Drawing for the job (mm, zero at the part's lowest x, y, z). Coordinates: 2 decimals unless noted, no trailing zeros. Write each loop counter-clockwise with the first axis right and the second up, starting at its lowest first coordinate (ties: lowest second). Pieces come first, ordered by that corner, then holes. Notation, with made-up numbers: (66, 87) -> (105, 87) arc R19 ccw to (105, 95) -> close; hole circle Ø1 at (-12, 22.5). An arc over 180 degrees is marked (long way). Write each question's results on one line, items separated by ' | '. Start each with the question number.
Q1. Drill centre lines: line 1 (Z direction, x = 23, y = 0.6); line 2 (Z direction, x = 22, y = 0.8). Where is each one in solid material? Low to high.
Q2. Saw through at A-A on z = 19. Give the cut face in (x, y).
Q3. Two-plate mould, pull along Y, no slides. Class the marked faces 1 and 2: released by +Y, released by -Y, zero draft, split by the parting line, or undercut.
Q4. Saw through at C-C on y = 0.2. Give the cut face in (x, z).
Q5. Saw through at B-B on x = 4. Give the cut face in (y, z).
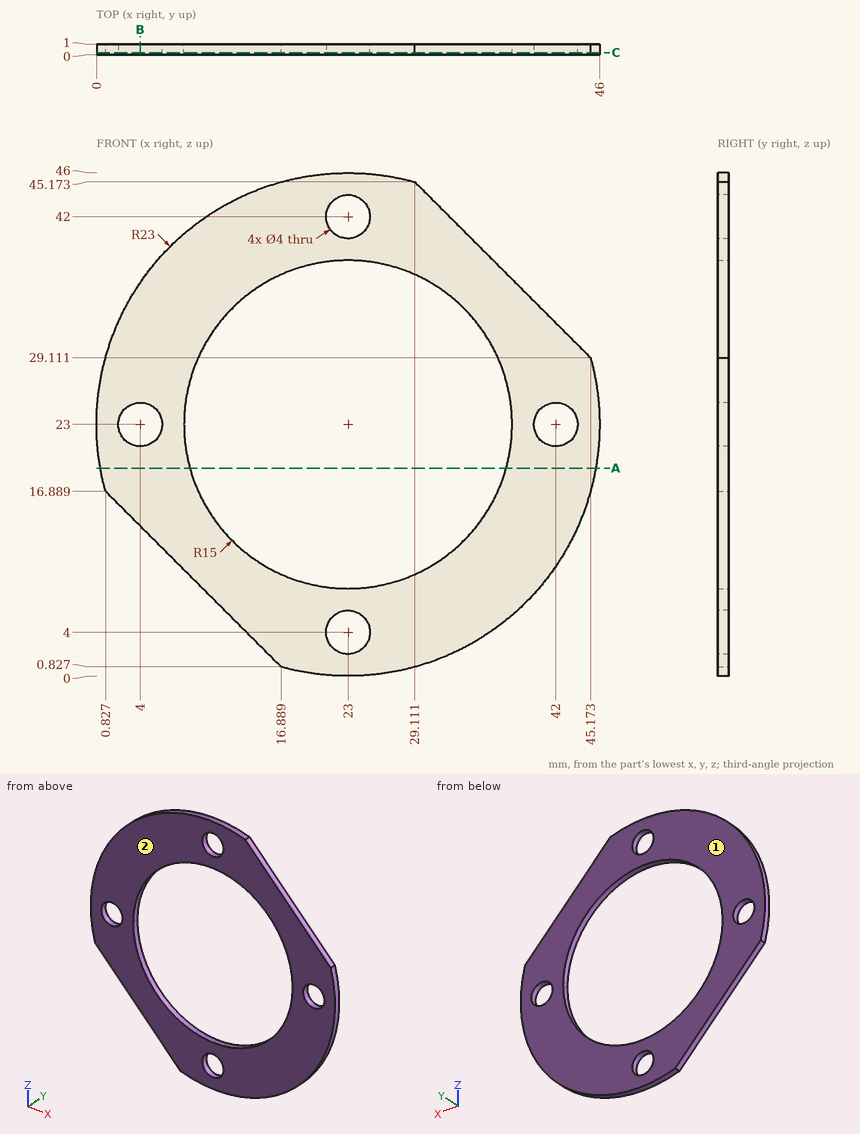
Returned:
1) line 1: z = 0 to 2, 6 to 8, 38 to 40, 44 to 46 | line 2: z = 0.02 to 2.27, 5.73 to 8.03, 37.97 to 40.27, 43.73 to 45.98
2) outline: (0.35, 0) -> (8.54, 0) -> (8.54, 1) -> (0.35, 1) -> close; (37.46, 0) -> (45.65, 0) -> (45.65, 1) -> (37.46, 1) -> close
3) face 1: released by +Y | face 2: released by -Y
4) outline: (0.83, 16.89) -> (16.89, 0.83) arc R23 ccw to (45.17, 29.11) -> (29.11, 45.17) arc R23 ccw to start; hole circle Ø4 at (4, 23); hole circle Ø30 at (23, 23); hole circle Ø4 at (23, 4); hole circle Ø4 at (23, 42); hole circle Ø4 at (42, 23)
5) outline: (0, 13.72) -> (1, 13.72) -> (1, 21) -> (0, 21) -> close; (0, 25) -> (1, 25) -> (1, 35.96) -> (0, 35.96) -> close
